```python
from build123d import *

# Parameters (mm, degrees)
SKETCH4_R          = 2.286
CUT_EXTRUDE1_DEPTH = 112.474173134


with BuildPart() as part:
    # Sketch3 → Revolve1 (revolve)
    with BuildSketch(Plane(origin=(0, 0, 0), x_dir=(0, 0, -1), z_dir=(1, 0, 0)), mode=Mode.PRIVATE) as revolve1_sk:
        with BuildLine():
            Line((0, 77.47), (0, 52.705))
            Line((0, 52.705), (0.635, 52.07))
            Line((0.635, 52.07), (1.524, 52.07))
            Line((1.524, 52.07), (1.524, 53.975))
            Line((1.524, 53.975), (20.574, 53.975))
            Line((20.574, 53.975), (20.574, 57.15))
            Line((20.574, 57.15), (8.89, 57.15))
            ThreePointArc((8.89, 57.15), (4.399871939, 59.009871939), (2.54, 63.5))
            Line((2.54, 63.5), (2.54, 77.47))
            Line((2.54, 77.47), (0, 77.47))
        make_face()
    revolve(revolve1_sk.sketch.rotate(Axis((0, 0, 0), (0, 0, -1)), 90), axis=Axis((0, 0, 0), (0, 0, -1)))

    # Sketch4 → Cut-Extrude1 (cut, through all)
    with BuildSketch(Plane.XY):
        with BuildLine():
            ThreePointArc((10.148016689, 76.802465177), (12.952013431, 75.713278366), (14.940104183, 73.455797294))
            Line((14.940104183, 73.455797294), (16.819480806, 69.871264453))
            ThreePointArc((16.819480806, 69.871264453), (18.384579854, 67.936367662), (20.573091868, 66.751557218))
            ThreePointArc((20.573091868, 66.751557218), (34.925, 60.491874454), (47.521998359, 51.192598801))
            ThreePointArc((47.521998359, 51.192598801), (49.642330309, 49.889697022), (52.100549608, 49.501729883))
            Line((52.100549608, 49.501729883), (56.14453442, 49.666408405))
            ThreePointArc((56.14453442, 49.666408405), (59.093615754, 49.073411844), (61.438877572, 47.189672839))
            ThreePointArc((61.438877572, 47.189672839), (38.735, 67.090988031), (10.148016689, 76.802465177))
        make_face()
        with BuildLine():
            ThreePointArc((-14.940104183, 73.455797294), (-12.952013431, 75.713278366), (-10.148016689, 76.802465177))
            ThreePointArc((-10.148016689, 76.802465177), (-38.735, 67.090988031), (-61.438877572, 47.189672839))
            ThreePointArc((-61.438877572, 47.189672839), (-59.093615754, 49.073411844), (-56.14453442, 49.666408405))
            Line((-56.14453442, 49.666408405), (-52.100549608, 49.501729883))
            ThreePointArc((-52.100549608, 49.501729883), (-49.642330309, 49.889697022), (-47.521998359, 51.192598801))
            ThreePointArc((-47.521998359, 51.192598801), (-34.925, 60.491874454), (-20.573091868, 66.751557218))
            ThreePointArc((-20.573091868, 66.751557218), (-18.384579854, 67.936367662), (-16.819480806, 69.871264453))
            Line((-16.819480806, 69.871264453), (-14.940104183, 73.455797294))
        make_face()
        with BuildLine():
            ThreePointArc((71.586894261, -29.612792338), (77.47, 0), (71.586894261, 29.612792338))
            ThreePointArc((71.586894261, 29.612792338), (72.045629184, 26.639866522), (71.084638604, 23.789388889))
            Line((71.084638604, 23.789388889), (68.920030414, 20.36953457))
            ThreePointArc((68.920030414, 20.36953457), (68.026910163, 18.04667064), (68.095090227, 15.558958417))
            ThreePointArc((68.095090227, 15.558958417), (69.85, 0), (68.095090227, -15.558958417))
            ThreePointArc((68.095090227, -15.558958417), (68.026910163, -18.04667064), (68.920030414, -20.36953457))
            Line((68.920030414, -20.36953457), (71.084638604, -23.789388889))
            ThreePointArc((71.084638604, -23.789388889), (72.045629184, -26.639866522), (71.586894261, -29.612792338))
        make_face()
        with BuildLine():
            ThreePointArc((-71.084638604, 23.789388889), (-72.045629184, 26.639866522), (-71.586894261, 29.612792338))
            ThreePointArc((-71.586894261, 29.612792338), (-77.47, 0), (-71.586894261, -29.612792338))
            ThreePointArc((-71.586894261, -29.612792338), (-72.045629184, -26.639866522), (-71.084638604, -23.789388889))
            Line((-71.084638604, -23.789388889), (-68.920030414, -20.36953457))
            ThreePointArc((-68.920030414, -20.36953457), (-68.026910163, -18.04667064), (-68.095090227, -15.558958417))
            ThreePointArc((-68.095090227, -15.558958417), (-69.85, 0), (-68.095090227, 15.558958417))
            ThreePointArc((-68.095090227, 15.558958417), (-68.026910163, 18.04667064), (-68.920030414, 20.36953457))
            Line((-68.920030414, 20.36953457), (-71.084638604, 23.789388889))
        make_face()
        with BuildLine():
            ThreePointArc((10.148016689, -76.802465177), (38.735, -67.090988031), (61.438877572, -47.189672839))
            ThreePointArc((61.438877572, -47.189672839), (59.093615754, -49.073411844), (56.14453442, -49.666408405))
            Line((56.14453442, -49.666408405), (52.100549608, -49.501729883))
            ThreePointArc((52.100549608, -49.501729883), (49.642330309, -49.889697022), (47.521998359, -51.192598801))
            ThreePointArc((47.521998359, -51.192598801), (34.925, -60.491874454), (20.573091868, -66.751557218))
            ThreePointArc((20.573091868, -66.751557218), (18.384579854, -67.936367662), (16.819480806, -69.871264453))
            Line((16.819480806, -69.871264453), (14.940104183, -73.455797294))
            ThreePointArc((14.940104183, -73.455797294), (12.952013431, -75.713278366), (10.148016689, -76.802465177))
        make_face()
        with BuildLine():
            ThreePointArc((-56.14453442, -49.666408405), (-59.093615754, -49.073411844), (-61.438877572, -47.189672839))
            ThreePointArc((-61.438877572, -47.189672839), (-38.735, -67.090988031), (-10.148016689, -76.802465177))
            ThreePointArc((-10.148016689, -76.802465177), (-12.952013431, -75.713278366), (-14.940104183, -73.455797294))
            Line((-14.940104183, -73.455797294), (-16.819480806, -69.871264453))
            ThreePointArc((-16.819480806, -69.871264453), (-18.384579854, -67.936367662), (-20.573091868, -66.751557218))
            ThreePointArc((-20.573091868, -66.751557218), (-34.925, -60.491874454), (-47.521998359, -51.192598801))
            ThreePointArc((-47.521998359, -51.192598801), (-49.642330309, -49.889697022), (-52.100549608, -49.501729883))
            Line((-52.100549608, -49.501729883), (-56.14453442, -49.666408405))
        make_face()
        with Locations((0, 73.025)):
            Circle(SKETCH4_R)
        with Locations((63.241505111, 36.5125)):
            Circle(SKETCH4_R)
        with Locations((63.241505111, -36.5125)):
            Circle(SKETCH4_R)
        with Locations((0, -73.025)):
            Circle(SKETCH4_R)
        with Locations((-63.241505111, -36.5125)):
            Circle(SKETCH4_R)
        with Locations((-63.241505111, 36.5125)):
            Circle(SKETCH4_R)
    extrude(amount=-CUT_EXTRUDE1_DEPTH, mode=Mode.SUBTRACT)


solid = part.part
```
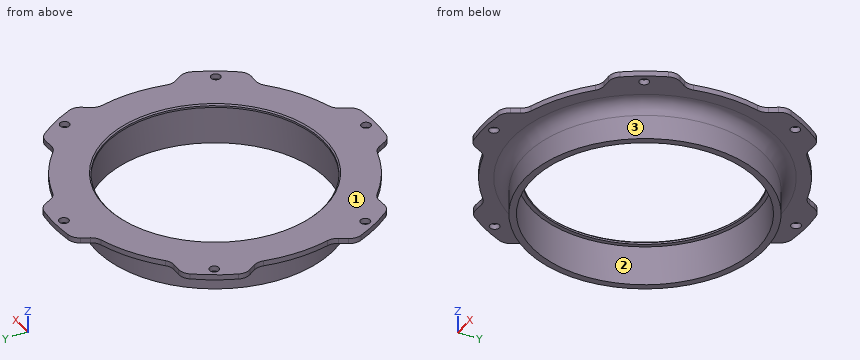
Can you work these out from the model? Positions are in its coordinate system, mm. Face numbers are marked on the shaded views. Give positions to 0.01 mm unless a question says otherwise; leave off trailing zeros. Loops run counter-clockwise (first coordinate to the right, second up) from the corner with the lowest first, then second, coordinate; pieces in that order, holes last. Notation, with made-up numbers: M 39,73 L 66,73 A12 ccw 66,90 Z; hole C 20,63 d5. An arc over 180 degrees is marked long. One line per item, written item: value.
(1) Suppose I cut it at A-A on x = 0. List the corners of the cut face in (y, z) for me (3 decimals), plus the area to 3 significant figures.
Returned:
outline: M -77.47,-2.54 L -75.311,-2.54 L -75.311,0 L -77.47,0 Z; M -70.739,-2.54 L -63.5,-2.54 A6.35 cw -57.15,-8.89 L -57.15,-20.574 L -53.975,-20.574 L -53.975,-1.524 L -52.07,-1.524 L -52.07,-0.635 L -52.705,0 L -70.739,0 Z; M 52.07,-1.524 L 53.975,-1.524 L 53.975,-20.574 L 57.15,-20.574 L 57.15,-8.89 A6.35 cw 63.5,-2.54 L 70.739,-2.54 L 70.739,0 L 52.705,0 L 52.07,-0.635 Z; M 75.311,-2.54 L 77.47,-2.54 L 77.47,0 L 75.311,0 Z
area: 233 mm^2
(2) Suppose I cut it at C-C on z = -16. List the corners of the cut face in (x, y) for me (3 decimals).
Returned:
outline: C 0,0 d114.3; hole C 0,0 d107.95
(3) Will these pins go through, and if not, where does the flat tip stop? pin 1 (12 mm diameter, centred on y = -50.5, z = -11, fed in from +X); pin 2 (8 mm diameter, centred on x = -42, z = -3.5, fed in from -Y); pin 3 (2 mm diameter, centred on x = -54, y = 35.5, fed in from -Z).
Returned:
pin 1: x = 35.86
pin 2: y = -58.53
pin 3: z = -2.54
(4) Suppose I cut it at B-B on y = 0. List the corners of the cut face in (x, z) for me (3 decimals), plus the area to 3 significant figures.
Returned:
outline: M -69.85,-2.54 L -63.5,-2.54 A6.35 cw -57.15,-8.89 L -57.15,-20.574 L -53.975,-20.574 L -53.975,-1.524 L -52.07,-1.524 L -52.07,-0.635 L -52.705,0 L -69.85,0 Z; M 52.07,-1.524 L 53.975,-1.524 L 53.975,-20.574 L 57.15,-20.574 L 57.15,-8.89 A6.35 cw 63.5,-2.54 L 69.85,-2.54 L 69.85,0 L 52.705,0 L 52.07,-0.635 Z
area: 218 mm^2
(5) I need wall thicknesses on line 1 (Y direction, x = 0, z = -1.05); line 2 (Y direction, x = 0, z = -15.25) (3 decimals); line 3 (X direction, y = -2, z = -15.5) (3 decimals). Which ranges of each line are inside material? Lowest first, please.
Returned:
line 1: -77.47 to -75.31, -70.74 to -52.07, 52.07 to 70.74, 75.31 to 77.47
line 2: -57.15 to -53.975, 53.975 to 57.15
line 3: -57.115 to -53.938, 53.938 to 57.115
(6) We'd pull the mould along Y, two halves only. Please class the marked faces 1, 2 and 3: released by +Y, released by -Y, zero draft, split by the parting line, or undercut.
Returned:
face 1: zero draft
face 2: undercut
face 3: split by the parting line
